from build123d import *

# Parameters (mm, degrees)
SKETCH1_R           = 3.5
BOSS_EXTRUDE1_DEPTH = 3.8
BOSS_EXTRUDE2_DEPTH = 1.4
SKETCH3_R           = 2.25
CUT_EXTRUDE1_DEPTH  = 2


with BuildPart() as part:
    # Sketch1 → Boss-Extrude1 (new body)
    with BuildSketch(Plane(origin=(0, 0, 0), x_dir=(1, 0, 0), z_dir=(0, 1, 0))):
        with Locations(Location((0, 0, 0), (0, 0, 90))):
            Circle(SKETCH1_R)
    extrude(amount=BOSS_EXTRUDE1_DEPTH)

    # Sketch2 → Boss-Extrude2 (add)
    with BuildSketch(Plane.XZ):
        with BuildLine():
            Line((-2, 14.192474485), (-2.625, 2.315032397))
            ThreePointArc((-2.625, 2.315032397), (0, 3.5), (2.625, 2.315032397))
            Line((2.625, 2.315032397), (2, 14.192474485))
            ThreePointArc((2, 14.192474485), (0, 16.09), (-2, 14.192474485))
        make_face()
    extrude(amount=-BOSS_EXTRUDE2_DEPTH)

    # Sketch3 → Cut-Extrude1 (cut)
    with BuildSketch(Plane(origin=(0, 3.8, 0), x_dir=(1, 0, 0), z_dir=(0, 1, 0))):
        with Locations(Location((0, 0, 0), (0, 0, 270))):
            Circle(SKETCH3_R)
    extrude(amount=-CUT_EXTRUDE1_DEPTH, mode=Mode.SUBTRACT)


solid = part.part
Design review of the part built by this model. Coordinates are the model's own, in mm. A direction names the side the tool comes from. Round coordinates to 2 decimals unless told otherwise and drop trailing zeros. Write each loop counter-clockwise with the first axis right and the second up, starting at its lowest first coordinate (ties: lowest second). Pieces come first, ordered by that corner, then holes. Notation, with made-up numbers: (37.5, -26.75) - (66.5, -26.75) arc R31 cw to (66.5, 6.25) - close; hole circle Ø6 at (-34.75, 81). An arc over 180 degrees is marked (long way). Use a Markdown table: item, result. Add a question column.
1. We need section A-A (x = 0). State the section outline as (y, z) points, then the cut area to 3 significant figures.
2. Wall thickness on probe 1 along X at (y, z) = (3.3, 0); probe 2 along Y at (x, z) = (-1.75, 1.25); probe 3 along Z at (x, y) = (2, 2.9): over which ranges is each line inside the solid? List them lowest first.
3. We need section B-B (z = 0). State the section outline as (x, y) points, then the cut area to 3 significant figures.
4. Clearance check with flat-ended pins moving along their axes: pin 1 (1.6 mm diameter, centred on x = -0.5, z = 6.5, fed in from +Y); pin 2 (2 mm diameter, centred on x = 0.5, z = -0.5, fed in from +Y). State where each tip first meets the part, or that it passes through.
5. Mouldability with a two-part tool opening along X and no side actions: class faces 1 (the face through (0.04, 0.69, 16.09)), 2 (the face through (0.676, 2.814, 2.146)), 3 (the face through (-2.308, 0.69, 8.337)) as +X half, -X half, draft (parallel to the pull), parting line (faces both ways), or undercut.
6. For faces 4 (the face through (0, 1.8, 0)), 5 (the face through (2.3, 3.8, -0.7)), list the 3-axis set-ups (+Z, -Z, +X, -X, +Y, -Y) from which the entire face can be reached by the end or side of a thin tool; tool diameter is ignored.
7. We need section D-D (x = -1.5). State the section outline as (y, z) points.
8. We need section C-C (y = 2.8). State the section outline as (x, z) points, then the cut area to 3 significant figures.
Output:
| question | item | result |
|---|---|---|
| 1 | outline | (0, -3.5) - (3.8, -3.5) - (3.8, -2.25) - (1.8, -2.25) - (1.8, 2.25) - (3.8, 2.25) - (3.8, 3.5) - (1.4, 3.5) - (1.4, 16.09) - (0, 16.09) - close |
| 1 | area | 35.2 mm2 |
| 2 | probe 1 | x = -3.5 to -2.25, 2.25 to 3.5 |
| 2 | probe 2 | y = 0 to 1.8 |
| 2 | probe 3 | z = -2.87 to -1.03, 1.03 to 2.87 |
| 3 | outline | (-3.5, 0) - (3.5, 0) - (3.5, 3.8) - (2.25, 3.8) - (2.25, 1.8) - (-2.25, 1.8) - (-2.25, 3.8) - (-3.5, 3.8) - close |
| 3 | area | 17.6 mm2 |
| 4 | pin 1 | stops at y = 1.4 |
| 4 | pin 2 | stops at y = 1.8 |
| 5 | face 1 | parting line |
| 5 | face 2 | undercut |
| 5 | face 3 | -X half |
| 6 | face 4 | +Y |
| 6 | face 5 | +Z, -Z, +X, -X, +Y |
| 7 | outline | (0, -3.16) - (3.8, -3.16) - (3.8, -1.68) - (1.8, -1.68) - (1.8, 1.68) - (3.8, 1.68) - (3.8, 3.16) - (1.4, 3.16) - (1.4, 15.41) - (0, 15.41) - close |
| 8 | outline | circle Ø7 at (0, 0); hole circle Ø4.5 at (0, 0) |
| 8 | area | 22.6 mm2 |
